Here's how the part is built. I have some questions about the finished solid (model axes, mm). A direction names the side the tool comes from. Give positions to 0.01 mm unless a question says otherwise; leave off trailing zeros. Order: outer loops, then holes, each group sorted by start corner. A loop starts at its lowest first (then second) coordinate and runs counter-clockwise, first axis right, second up.
from build123d import *

# Parameters (mm, degrees)
SKETCH1_W           = 70
SKETCH1_H           = 25
BOSS_EXTRUDE1_DEPTH = 5
SKETCH2_R           = 1.25
CUT_EXTRUDE2_DEPTH  = 6
SKETCH5_W           = 10
SKETCH5_H           = 25
BOSS_EXTRUDE3_DEPTH = 20
FILLET1_R           = 10
SKETCH6_R           = 1.7
CUT_EXTRUDE3_DEPTH  = 11


with BuildPart() as part:
    # Sketch1 → Boss-Extrude1 (new body)
    with BuildSketch(Plane.XY):
        with Locations((35, -12.5)):
            Rectangle(SKETCH1_W, SKETCH1_H)
    extrude(amount=BOSS_EXTRUDE1_DEPTH)

    # Sketch2 → Cut-Extrude2 (cut, through all)
    with BuildSketch(Plane.XY.offset(5)):
        with Locations((41, -2)):
            Circle(SKETCH2_R)
        with Locations((59, -2)):
            Circle(SKETCH2_R)
    extrude(amount=-CUT_EXTRUDE2_DEPTH, mode=Mode.SUBTRACT)

    # Sketch5 → Boss-Extrude3 (add)
    with BuildSketch(Plane.XY.offset(5)):
        with Locations((5, -12.5)):
            Rectangle(SKETCH5_W, SKETCH5_H)
    extrude(amount=BOSS_EXTRUDE3_DEPTH)

    # Fillet1
    fillet1_edges = [part.edges().sort_by_distance(p)[0] for p in [
        (10, -12.5, 5),
    ]]
    fillet(fillet1_edges, radius=FILLET1_R)

    # Sketch6 → Cut-Extrude3 (cut, through all)
    with BuildSketch(Plane(origin=(10, 0, 0), x_dir=(0, 0, -1), z_dir=(1, 0, 0))):
        with Locations((-20, -21.834919238)):
            Circle(SKETCH6_R)
        with Locations((-20, -5.503108416)):
            Circle(SKETCH6_R)
    extrude(amount=-CUT_EXTRUDE3_DEPTH, mode=Mode.SUBTRACT)


solid = part.part
Q1. For faces 4 (the face through (5.07, -23.343, 19.216)), 5 (the face through (10, -13, 20)), which set-ups out of +Z, -Z, +X, -X, +Y, -Y let a thin tool reach every point of the face, with its end or its side?
Filled sheet:
face 4: +X, -X
face 5: +Z, +X, +Y, -Y
Q2. I'm going to push flat-ended pins straight in: P1, Ø4, axis at y = -13, z = 5.5, coming from the -X side; P2, Ø2, axis at y = -5.5, z = 20, coming from the +X side; P3, Ø4, axis at x = 41, y = -2, coming from the +Z side; P4, Ø4, axis at y = -21.5, z = 15, coming from the +X side. Where does each tip first touch, or does it pass through?
Filled sheet:
P1: stops at x = 0
P2: passes through
P3: stops at z = 5
P4: stops at x = 10.2
Q3. If we section it at D-D on z = 23.5: List the corners of the cut face in (x, y) for me, plus the area to 3 significant figures.
Filled sheet:
outline: (0, -25) - (10, -25) - (10, 0) - (0, 0) - close
area: 250 mm2
Q4. I need wall thicknesses on L1, parallel to Y at x = 7.25, z = 20; L2, parallel to X at y = -9.5, z = 19.5; L3, parallel to Z at x = 40, y = -17.25. Which ranges of each line are inside material? Lowest first, please.
Filled sheet:
L1: y = -25 to -23.53, -20.13 to -7.2, -3.8 to 0
L2: x = 0 to 10
L3: z = 0 to 5
Q5. Thinking about a two-plate mould opening in Y: for faces 1 (the face through (22, -25, 4)), 2 (the face through (5, -12, 25)), 3 (the face through (39.75, -1.95, 2.54)), which applies, released by +Y, released by -Y, zero draft, split by the parting line, or undercut?
Filled sheet:
face 1: released by -Y
face 2: zero draft
face 3: undercut
Q6. If we section it at C-C on x = 5.5: List the corners of the cut face in (y, z) for me, plus the area to 3 significant figures.
Filled sheet:
outline: (-25, 0) - (0, 0) - (0, 25) - (-25, 25) - close; hole circle Ø3.4 at (-21.83, 20); hole circle Ø3.4 at (-5.5, 20)
area: 607 mm2
Q7. If we section it at B-B on x = 59: List the corners of the cut face in (y, z) for me.
Filled sheet:
outline: (-25, 0) - (-3.25, 0) - (-3.25, 5) - (-25, 5) - close; (-0.75, 0) - (0, 0) - (0, 5) - (-0.75, 5) - close
Q8. If we section it at A-A on y = -13.75: List the corners of the cut face in (x, z) for me.
Filled sheet:
outline: (0, 0) - (70, 0) - (70, 5) - (20, 5) arc R10 cw to (10, 15) - (10, 25) - (0, 25) - close
